Geometry: final body of the model. Coordinates: model frame, mm. A direction names the side the tool comes from. Coordinates: 2 decimals unless noted, no trailing zeros. Order: outer loops, then holes, each group sorted by start corner. A loop starts at its lowest first (then second) coordinate and runs counter-clockwise, first axis right, second up. Notation, with made-up numbers: (85.25, -26) -> (114.25, -26) arc R14 ccw to (114.25, -15) -> close; hole circle Ø7 at (89.25, 70.25). An arc over 180 degrees is marked (long way). Use one line per item in the form item = value.
```python
from build123d import *

# Parameters (mm, degrees)
PAD_DEPTH     = 3
SKETCH002_R   = 1.5
POCKET_DEPTH  = 3.001
SKETCH001_R   = 3
SKETCH001_R_2 = 1.5
PAD001_DEPTH  = 28
FILLET_R      = 0.5


with BuildPart() as part:
    # Sketch → Pad (new body)
    with BuildSketch(Plane.XY):
        Polygon((-7.8, 27), (42.8, 27), (42.8, -27), (18.3, -27), (18.3, -4), (13.3, -4), (13.3, -27), (-42.8, -27), (-42.8, 21), (-7.8, 21), align=None)
    extrude(amount=PAD_DEPTH)

    # Sketch002 → Pocket (cut, through all)
    with BuildSketch(Plane.XY.offset(3)):
        with Locations((1.2, 23)):
            Circle(SKETCH002_R)
        with Locations((9.2, 23)):
            Circle(SKETCH002_R)
        with Locations((17.2, 23)):
            Circle(SKETCH002_R)
        with Locations((25.2, 23)):
            Circle(SKETCH002_R)
        with Locations((33.2, 23)):
            Circle(SKETCH002_R)
        with Locations((-38.8, 15)):
            Circle(SKETCH002_R)
        with Locations((-30.8, 15)):
            Circle(SKETCH002_R)
        with Locations((-22.8, 15)):
            Circle(SKETCH002_R)
        with Locations((-14.8, 15)):
            Circle(SKETCH002_R)
        with Locations((-6.8, 15)):
            Circle(SKETCH002_R)
        with Locations((1.2, 15)):
            Circle(SKETCH002_R)
        with Locations((9.2, 15)):
            Circle(SKETCH002_R)
        with Locations((17.2, 15)):
            Circle(SKETCH002_R)
        with Locations((25.2, 15)):
            Circle(SKETCH002_R)
        with Locations((33.2, 15)):
            Circle(SKETCH002_R)
        with Locations((-38.8, 7)):
            Circle(SKETCH002_R)
        with Locations((-30.8, 7)):
            Circle(SKETCH002_R)
        with Locations((-22.8, 7)):
            Circle(SKETCH002_R)
        with Locations((-14.8, 7)):
            Circle(SKETCH002_R)
        with Locations((-6.8, 7)):
            Circle(SKETCH002_R)
        with Locations((1.2, 7)):
            Circle(SKETCH002_R)
        with Locations((9.2, 7)):
            Circle(SKETCH002_R)
        with Locations((17.2, 7)):
            Circle(SKETCH002_R)
        with Locations((25.2, 7)):
            Circle(SKETCH002_R)
        with Locations((33.2, 7)):
            Circle(SKETCH002_R)
        with Locations((-38.8, -1)):
            Circle(SKETCH002_R)
        with Locations((-30.8, -1)):
            Circle(SKETCH002_R)
        with Locations((-22.8, -1)):
            Circle(SKETCH002_R)
        with Locations((-14.8, -1)):
            Circle(SKETCH002_R)
        with Locations((-6.8, -1)):
            Circle(SKETCH002_R)
        with Locations((1.2, -1)):
            Circle(SKETCH002_R)
        with Locations((9.2, -1)):
            Circle(SKETCH002_R)
        with Locations((17.2, -1)):
            Circle(SKETCH002_R)
        with Locations((25.2, -1)):
            Circle(SKETCH002_R)
        with Locations((33.2, -1)):
            Circle(SKETCH002_R)
        with Locations((-38.8, -9)):
            Circle(SKETCH002_R)
        with Locations((-30.8, -9)):
            Circle(SKETCH002_R)
        with Locations((-22.8, -9)):
            Circle(SKETCH002_R)
        with Locations((-6.8, -9)):
            Circle(SKETCH002_R)
        with Locations((1.2, -9)):
            Circle(SKETCH002_R)
        with Locations((9.2, -9)):
            Circle(SKETCH002_R)
        with Locations((25.2, -9)):
            Circle(SKETCH002_R)
        with Locations((33.2, -9)):
            Circle(SKETCH002_R)
        with Locations((-38.8, -17)):
            Circle(SKETCH002_R)
        with Locations((-30.8, -17)):
            Circle(SKETCH002_R)
        with Locations((-22.8, -17)):
            Circle(SKETCH002_R)
        with Locations((-14.8, -17)):
            Circle(SKETCH002_R)
        with Locations((-6.8, -17)):
            Circle(SKETCH002_R)
        with Locations((1.2, -17)):
            Circle(SKETCH002_R)
        with Locations((9.2, -17)):
            Circle(SKETCH002_R)
        with Locations((25.2, -17)):
            Circle(SKETCH002_R)
        with Locations((33.2, -17)):
            Circle(SKETCH002_R)
    extrude(amount=-POCKET_DEPTH, mode=Mode.SUBTRACT)

    # Sketch001 → Pad001 (new body)
    with BuildSketch(Plane.XY.offset(3)):
        with Locations((-17.3, -9)):
            Circle(SKETCH001_R)
        with Locations((-17.3, -9)):
            Circle(SKETCH001_R_2, mode=Mode.SUBTRACT)
        with Locations((37.8, 14.5)):
            Circle(SKETCH001_R)
        with Locations((37.8, 14.5)):
            Circle(SKETCH001_R_2, mode=Mode.SUBTRACT)
    extrude(amount=-PAD001_DEPTH)

    # Fillet
    fillet_edges = [part.edges().sort_by_distance(p)[0] for p in [
        (34.8, 14.5, 0),
        (-20.3, -9, 0),
    ]]
    fillet(fillet_edges, radius=FILLET_R)


solid = part.part
```
1) Section B-B, the plane z = -8.25. Output: boundary loops of the cut face in (x, y), and give its area (3 significant figures).
Results found:
outline = circle Ø6 at (-17.3, -9); circle Ø6 at (37.8, 14.5); hole circle Ø3 at (-17.3, -9); hole circle Ø3 at (37.8, 14.5)
area = 42.4 mm2
2) Section D-D, the plane y = 23. Output: boundary loops of the cut face in (x, z), and give its area (3 significant figures).
Results found:
outline = (-7.8, 0) -> (-0.3, 0) -> (-0.3, 3) -> (-7.8, 3) -> close; (2.7, 0) -> (7.7, 0) -> (7.7, 3) -> (2.7, 3) -> close; (10.7, 0) -> (15.7, 0) -> (15.7, 3) -> (10.7, 3) -> close; (18.7, 0) -> (23.7, 0) -> (23.7, 3) -> (18.7, 3) -> close; (26.7, 0) -> (31.7, 0) -> (31.7, 3) -> (26.7, 3) -> close; (34.7, 0) -> (42.8, 0) -> (42.8, 3) -> (34.7, 3) -> close
area = 107 mm2
3) Pull-direction query (X, two-part tool) for faces 1 (the flat face through (31, -27, 1)), 2 (the cylindrical face through (40.57, 13.35, -12.49)), 3 (the cylindrical face through (23.7, -0.93, 1.52)); classes: released by +X, released by -X, zero draft, split by the parting line, or undercut.
Results found:
face_1 = zero draft
face_2 = split by the parting line
face_3 = undercut
4) Contact query for flat-ended pins moving along their axis: P1, Ø3.5, axis at x = 9.2, y = -17, coming from the -Z side; P2, Ø1.8, axis at x = 17.2, y = 15, coming from the -Z side. Output: stop coordinate, or through.
Results found:
P1 = 0
P2 = through
5) Access query for faces 4 (the cylindrical face through (8, -1.9, 1.5)), 5 (the cylindrical face through (-14.44, -8.1, -12.58)). Directions: +Z, -Z, +X, -X, +Y, -Y. A direction counts if a zero-diameter tool reaches every point of the face in a straight line with its end or side. Return the directions, or none.
Results found:
face_4 = +Z, -Z
face_5 = -Z
6) Material intervals for probe 1 along Y at (x, z) = (-22.8, 0.7); probe 2 along Z at (x, y) = (4.5, -20); probe 3 along Y at (x, z) = (-17.3, -19), sorted ascending. Write a range as from..to.
Results found:
probe_1 = -27..-18.5, -15.5..-10.5, -7.5..-2.5, 0.5..5.5, 8.5..13.5, 16.5..21
probe_2 = 0..3
probe_3 = -12..-10.5, -7.5..-6
7) Section C-C, the plane x = 1.2. Output: boundary loops of the cut face in (y, z), and give its area (3 significant figures).
Results found:
outline = (-27, 0) -> (-18.5, 0) -> (-18.5, 3) -> (-27, 3) -> close; (-15.5, 0) -> (-10.5, 0) -> (-10.5, 3) -> (-15.5, 3) -> close; (-7.5, 0) -> (-2.5, 0) -> (-2.5, 3) -> (-7.5, 3) -> close; (0.5, 0) -> (5.5, 0) -> (5.5, 3) -> (0.5, 3) -> close; (8.5, 0) -> (13.5, 0) -> (13.5, 3) -> (8.5, 3) -> close; (16.5, 0) -> (21.5, 0) -> (21.5, 3) -> (16.5, 3) -> close; (24.5, 0) -> (27, 0) -> (27, 3) -> (24.5, 3) -> close
area = 108 mm2
8) Section A-A, the plane x = 17.2. Output: boundary loops of the cut face in (y, z).
Results found:
outline = (-4, 0) -> (-2.5, 0) -> (-2.5, 3) -> (-4, 3) -> close; (0.5, 0) -> (5.5, 0) -> (5.5, 3) -> (0.5, 3) -> close; (8.5, 0) -> (13.5, 0) -> (13.5, 3) -> (8.5, 3) -> close; (16.5, 0) -> (21.5, 0) -> (21.5, 3) -> (16.5, 3) -> close; (24.5, 0) -> (27, 0) -> (27, 3) -> (24.5, 3) -> close
